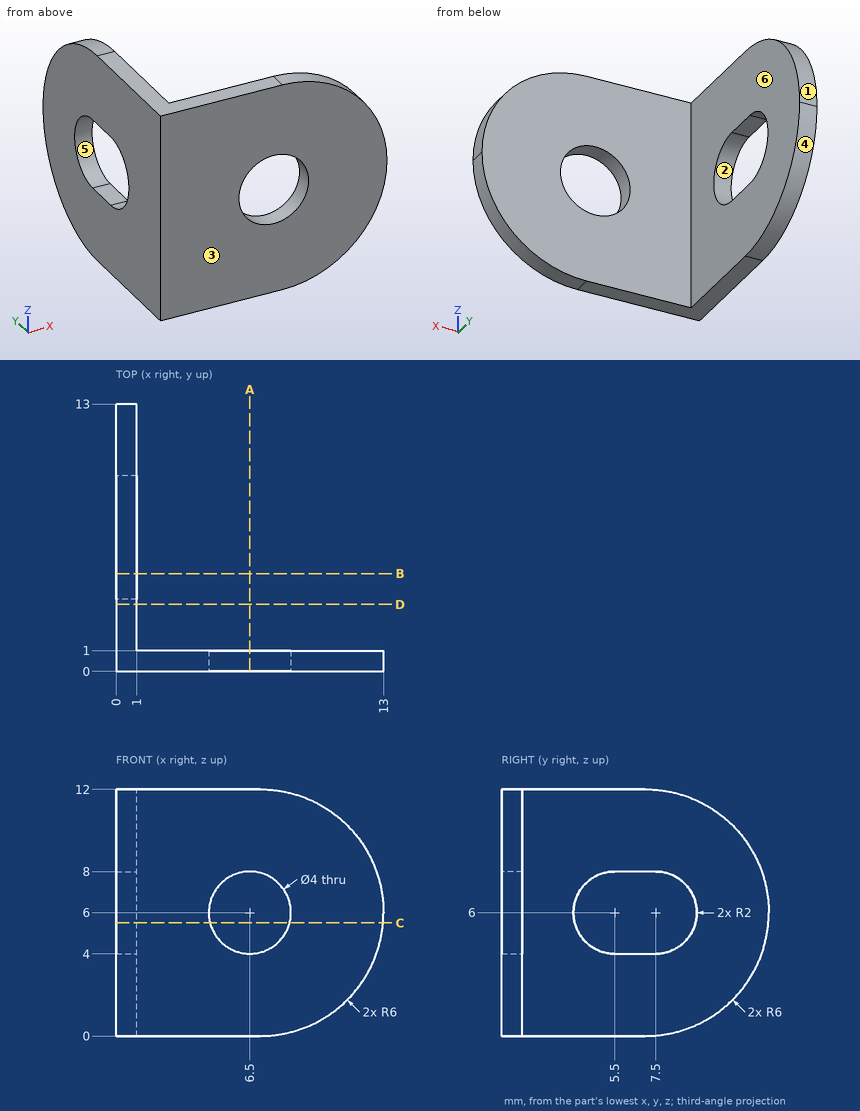
Answer from the drawing. Dimensions are ordinates in mm from the lowest x, y and z of the part. A direction names the side the tool comes from. Give positions to 0.01 mm unless a question says otherwise; leave off trailing zeros. Order: outer loops, then holes, each group sorted by start corner. A loop starts at its lowest first (then second) coordinate and runs counter-clockwise, first axis right, second up. Notation, with made-up numbers: (64.5, 40.25) - (74.5, 40.25) arc R29 ccw to (74.5, 74.25) - close; hole circle Ø9 at (29.25, -3). An arc over 180 degrees is marked (long way). One line per item, written item: value. Start each with the question number.
1) A cutting plane is placed at A-A on x = 6.5. Give the vertices of the cut face in (y, z), then the cut area to 3 significant figures.
2) The mould has two halves that part along Y. Classify the marked faces 1, 2 and 3: released by +Y, released by -Y, zero draft, split by the parting line, or undercut.
3) Given pin 1 Ø2 at (x, y) = (4, 3) entering from +Z; pin 2 Ø4 at (y, z) = (2, 3.5) entering from +X, each flat-ended and moving along its own axis, determine where each tip first touches the part or whether it passes through.
4) A cutting plane is placed at D-D on y = 3.25. Give the vertices of the cut face in (x, z).
5) Find the intervals of material crossed by L1, parallel to X at y = 0.6, z = 6; L2, parallel to Y at x = 5.25, z = 10, in increasing order.
6) A tool of negligible diameter and unlimited length cuts with its end or side. For the marked faces 4, 5 and 6, from which of +Z, -Z, +X, -X, +Y, -Y can it reach the whole face along a straight path? Write none if from no direction.
7) A cutting plane is placed at C-C on z = 5.5. Give the vertices of the cut face in (x, y), then the cut area to 3 significant figures.
8) A cutting plane is placed at B-B on y = 4.75. Give the vertices of the cut face in (x, z).
Answer sheet:
1. outline: (0, 0) - (1, 0) - (1, 4) - (0, 4) - close; (0, 8) - (1, 8) - (1, 12) - (0, 12) - close
1. area: 8.00 mm2
2. face 1: released by +Y
2. face 2: undercut
2. face 3: released by -Y
3. pin 1: passes through
3. pin 2: stops at x = 12.95
4. outline: (0, 0) - (1, 0) - (1, 12) - (0, 12) - close
5. L1: x = 0 to 4.5, 8.5 to 13
5. L2: y = 0 to 1
6. face 4: -Z, +X, -X, +Y
6. face 5: +X, -X
6. face 6: +Z, -Z, +X, +Y
7. outline: (0, 0) - (4.56, 0) - (4.56, 1) - (1, 1) - (1, 3.56) - (0, 3.56) - close; (0, 9.44) - (1, 9.44) - (1, 12.98) - (0, 12.98) - close; (8.44, 0) - (12.98, 0) - (12.98, 1) - (8.44, 1) - close
7. area: 15.2 mm2
8. outline: (0, 0) - (1, 0) - (1, 4.15) - (0, 4.15) - close; (0, 7.85) - (1, 7.85) - (1, 12) - (0, 12) - close
